```python
from build123d import *

# Parameters (mm, degrees)
F0_W     = 206.375
F0_H     = 15.875
F1_DEPTH = 38.1
F2_R     = 19.04999
F3_R     = 19.04999
F4_R     = 9.525
F5_DEPTH = 101.6
F6_R     = 9.525
F7_DEPTH = 25.4
F8_R     = 9.525
F9_DEPTH = 25.4


# Not quite as in the source:
# - a fillet or chamfer is up to 0.001 mm smaller than in the source, because OpenCascade refuses the exact size


with BuildPart() as f1:
    # F0 (on Front) → F1 (new body)
    with BuildSketch(Plane.XZ):
        with Locations((103.1875, -7.9375)):
            Rectangle(F0_W, F0_H)
    extrude(amount=F1_DEPTH)

    # F3 (radius 19.05 in the source; OpenCascade refuses exactly that, so slightly less here)
    f3_edges = [f1.edges().sort_by_distance(p)[0] for p in [
        (0, -38.1, -7.9375),
        (206.375, -38.1, -7.9375),
        (206.375, 0, -7.9375),
        (0, 0, -7.9375),
    ]]
    fillet(f3_edges, radius=F3_R)



with BuildPart() as f1b:
    # F0 (on Front) → F1, piece 2 (new body)
    with BuildSketch(Plane.XZ):
        with Locations((-65.0875, 109.5375)):
            Rectangle(F0_W, F0_H)
    extrude(amount=F1_DEPTH)

    # F2 (radius 19.05 in the source; OpenCascade refuses exactly that, so slightly less here)
    f2_edges = [f1b.edges().sort_by_distance(p)[0] for p in [
        (-168.275, -38.1, 109.5375),
        (-168.275, 0, 109.5375),
        (38.1, -38.1, 109.5375),
        (38.1, 0, 109.5375),
    ]]
    fillet(f2_edges, radius=F2_R)


with BuildPart() as f1_1:
    add(f1.part)

    add(f1b.part)  # F5 merges F1b
    # F4 (on face) → F5 (join)
    with BuildSketch(Plane(origin=(0, 0, 101.6), x_dir=(1, 0, 0), z_dir=(0, 0, -1))):
        with Locations((19.05, 19.05)):
            Circle(F4_R)
    extrude(amount=F5_DEPTH)

    # F6 (on face) → F7 (cut)
    with BuildSketch(Plane(origin=(0, 0, 101.6), x_dir=(1, 0, 0), z_dir=(0, 0, -1))):
        with Locations((-149.225, 19.05)):
            Circle(F6_R)
    extrude(amount=-F7_DEPTH, mode=Mode.SUBTRACT)

    # F8 (on face) → F9 (cut)
    with BuildSketch(Plane(origin=(0, 0, -15.875), x_dir=(1, 0, 0), z_dir=(0, 0, -1))):
        with Locations((187.325, 19.05)):
            Circle(F8_R)
    extrude(amount=-F9_DEPTH, mode=Mode.SUBTRACT)


solid = f1_1.part
```
The model under review builds one solid part; all positions refer to its coordinate system, in mm. A direction names the side the tool comes from. Coordinates: 2 decimals unless noted, no trailing zeros. Write each loop counter-clockwise with the first axis right and the second up, starting at its lowest first coordinate (ties: lowest second). Pieces come first, ordered by that corner, then holes. Notation, with made-up numbers: (-3.75, 27.5) -> (4.25, 27.5) arc R21 ccw to (4.25, 35.5) -> close; hole circle Ø4 at (10.5, -31). An arc over 180 degrees is marked (long way). One line per item, written item: value. Start each with the question number.
Q1. For faces 1 (the face through (16.99, -9.75, 51.51)), 2 (the face through (5.43, -32.37, -7.83)), 3 (the face through (32.67, -32.37, 109.65)), 4 (the face through (5.43, -5.73, -7.83)), 5 (the face through (32.67, -5.73, 109.65)), list the 3-axis set-ups (+Z, -Z, +X, -X, +Y, -Y) from which the entire face can be reached by the end or side of a thin tool; tool diameter is ignored.
Q2. Add section D-D, the plane x = -84. Give the boundary of the cut face in (y, z) (3 decimals), then the cut area to 3 significant figures.
Q3. Add section B-B, the plane z = 30.5. Give the boundary of the cut face in (x, y) (3 decimals).
Q4. Add section C-C, the plane y = -34. Give the boundary of the cut face in (x, z) (3 decimals), then the cut area to 3 significant figures.
Q5. To check wall thickness, follow probe 1 along X at (y, z) = (-15, -3); probe 2 along Z at (x, y) = (-121, -12) (3 decimals); probe 3 along Z at (x, y) = (59, -31) (3 decimals). State the ranges of each line that lie inside material, in increasing order.
Q6. Clearance check with flat-ended pins moving along their axes: P1, Ø6, axis at x = -99, y = -24, coming from the -Z side; P2, Ø4, axis at y = -28.5, z = 91.5, coming from the +X side; P3, Ø6, axis at y = -29, z = 24.5, coming from the +X side. State where each tip first meets the part, or that it passes through.
Q7. The part is to be moulded in two halves that separate along Y. For faces 6 (the face through (-140.426, -15.402, 109.426)), 7 (the face through (-66, 0, 110)), 8 (the face through (102, -19, 0)), say which applies: +Y half, -Y half, draft (parallel to the pull), parting line (faces both ways), or undercut.
Q8. Add section A-A, the plane y = -4.5. Give the boundary of the cut face in (x, z) (3 decimals), then the cut area to 3 significant figures.
Response:
1. face 1: none
1. face 2: -Z, -X, -Y
1. face 3: +Z, +X, -Y
1. face 4: -Z, -X, +Y
1. face 5: +Z, +X, +Y
2. outline: (-38.1, 101.6) -> (0, 101.6) -> (0, 117.475) -> (-38.1, 117.475) -> close
2. area: 605 mm²
3. outline: circle Ø19.05 at (19.05, -19.05)
4. outline: (-161.032, 101.6) -> (30.857, 101.6) -> (30.857, 117.475) -> (-161.032, 117.475) -> close; (7.243, -15.875) -> (199.132, -15.875) -> (199.132, 0) -> (7.243, 0) -> close
4. area: 6,090 mm²
5. probe 1: 0.44 to 178.7, 195.95 to 205.94
5. probe 2: 101.6 to 117.475
5. probe 3: -15.875 to 0
6. P1: z = 101.6
6. P2: x = 24.98
6. P3: x = 25.56
7. face 6: undercut
7. face 7: +Y half
7. face 8: draft
8. outline: (-161.521, 101.6) -> (31.346, 101.6) -> (31.346, 117.475) -> (-161.521, 117.475) -> close; (6.754, -15.875) -> (199.621, -15.875) -> (199.621, 0) -> (6.754, 0) -> close
8. area: 6,120 mm²
